CAD build for the part. Positions are in the model's coordinates, mm. Give positions to 0.01 mm unless a question says otherwise; leave off trailing zeros. Put each result on its own line as item: value. Start each with the question number.
1. Drop a flat-ended pin along its axis: pin 1 (2 mm diameter, centred on x = -42, z = 4.5, fed in from -Y). Give the stop position or say it passes through.
2. Wall check: line 1 (Y direction, x = -19, z = 5.25); line 2 (Y direction, x = -62, z = 2); line 3 (X direction, y = -12, z = 4.5). Give the ranges that are in metal, low to high.
3. Cut at A-A on z = 3. Give the number of separate pieces and of enclosed holes in the cut face, and give its area (3 significant figures).
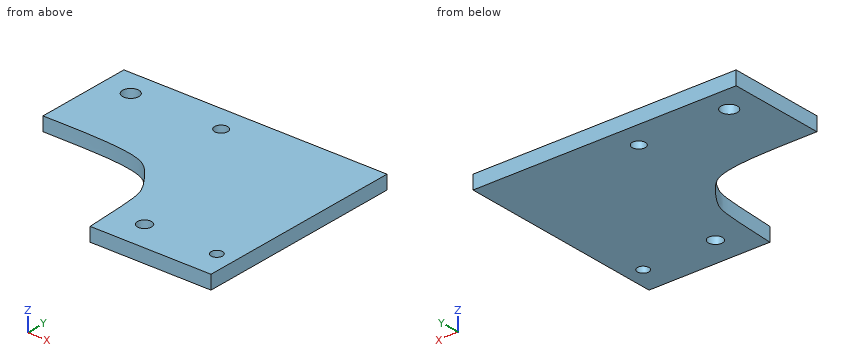
from build123d import *

# Parameters (mm, degrees)
F0_R     = 3.227705
F0_R_2   = 2.6202831703
F0_R_3   = 3.7211
F0_R_4   = 3.0099
F1_DEPTH = 6.35


with BuildPart() as f1:
    # F0 (on Top) → F1 (new body)
    with BuildSketch(Plane.XY):
        with BuildLine():
            Line((50.3533543698, 50.5695272586), (-70.2966456302, 50.5695272586))
            Line((-70.2966456302, 50.5695272586), (-70.2966456302, 6.1389088832))
            add(Edge.make_bspline(
                [(-70.2966456302, 6.1389088832), (-52.0441571305, 6.2243048177), (-24.7506450339, 6.3520000068), (-16.0268583665, -2.7376199674), (-8.2325781541, -12.9339469203), (-6.413955806, -21.4539728098), (-5.5948416135, -36.5589979729), (-5.0773202083, -46.1024461493)],
                knots=[0, 0, 0, 0, 0.3147391889, 0.4706392699, 0.6307003445, 0.7666741971, 1, 1, 1, 1], degree=3))
            Line((-5.0773202083, -46.1024461493), (50.3533543698, -46.1024461493))
            Line((50.3533543698, -46.1024461493), (50.3533543698, 50.5695272586))
        make_face()
        with Locations((8.6481217295, -32.6273292303)):
            Circle(F0_R, mode=Mode.SUBTRACT)
        with Locations((42.2276780009, -33.1594906747)):
            Circle(F0_R_2, mode=Mode.SUBTRACT)
        with Locations((-57.2580881417, 38.7286692858)):
            Circle(F0_R_3, mode=Mode.SUBTRACT)
        with Locations((-15.8467981964, 38.7890487909)):
            Circle(F0_R_4, mode=Mode.SUBTRACT)
    extrude(amount=F1_DEPTH)


solid = f1.part
Report:
1. pin 1: stops at y = 5.72
2. line 1: y = 0.05 to 50.57
2. line 2: y = 6.17 to 50.57
2. line 3: x = -9.51 to 50.35
3. separate pieces: 1
3. enclosed holes: 4
3. area: 8,410 mm²
